For this review, take the finished solid that the model builds, in its own axes (mm). A direction names the side the tool comes from. Give positions to 0.01 mm unless a question says otherwise; leave off trailing zeros. Put each result on its own line as item: value. Start each with the question number.
from build123d import *

# Parameters (mm, degrees)
EXTRUDE_1_DEPTH                     = 401.066
SKETCH_2_R                          = 7.1501
CUT_EXTRUDE_1_DEPTH                 = 5.08
PATTERN_LINEAR_1_COUNT              = 8
PATTERN_LINEAR_1_PITCH              = 47.752
PATTERN_CIRCULAR_2_COUNT            = 3
PATTERN_CIRCULAR_2_ANGLE            = 180
PATTERN_CIRCULAR_2_COPY_1_SKETCH_R  = 7.1501
PATTERN_CIRCULAR_2_COPY_1_DEPTH     = 5.08
PATTERN_CIRCULAR_2_COPY_2_SKETCH_R  = 7.1501
PATTERN_CIRCULAR_2_COPY_2_DEPTH     = 5.08
PATTERN_CIRCULAR_2_COPY_3_SKETCH_R  = 7.1501
PATTERN_CIRCULAR_2_COPY_3_DEPTH     = 5.08
PATTERN_CIRCULAR_2_COPY_4_SKETCH_R  = 7.1501
PATTERN_CIRCULAR_2_COPY_4_DEPTH     = 5.08
PATTERN_CIRCULAR_2_COPY_5_SKETCH_R  = 7.1501
PATTERN_CIRCULAR_2_COPY_5_DEPTH     = 5.08
PATTERN_CIRCULAR_2_COPY_6_SKETCH_R  = 7.1501
PATTERN_CIRCULAR_2_COPY_6_DEPTH     = 5.08
PATTERN_CIRCULAR_2_COPY_7_SKETCH_R  = 7.1501
PATTERN_CIRCULAR_2_COPY_7_DEPTH     = 5.08
PATTERN_CIRCULAR_2_COPY_8_SKETCH_R  = 7.1501
PATTERN_CIRCULAR_2_COPY_8_DEPTH     = 5.08
PATTERN_CIRCULAR_2_COPY_9_SKETCH_R  = 7.1501
PATTERN_CIRCULAR_2_COPY_9_DEPTH     = 5.08
PATTERN_CIRCULAR_2_COPY_10_SKETCH_R = 7.1501
PATTERN_CIRCULAR_2_COPY_10_DEPTH    = 5.08
PATTERN_CIRCULAR_2_COPY_11_SKETCH_R = 7.1501
PATTERN_CIRCULAR_2_COPY_11_DEPTH    = 5.08
PATTERN_CIRCULAR_2_COPY_12_SKETCH_R = 7.1501
PATTERN_CIRCULAR_2_COPY_12_DEPTH    = 5.08
PATTERN_CIRCULAR_2_COPY_13_SKETCH_R = 7.1501
PATTERN_CIRCULAR_2_COPY_13_DEPTH    = 5.08
PATTERN_CIRCULAR_2_COPY_14_SKETCH_R = 7.1501
PATTERN_CIRCULAR_2_COPY_14_DEPTH    = 5.08


with BuildPart() as part:
    # 草图1 → 凸台-拉伸1 (new body)
    with BuildSketch(Plane.XY):
        with BuildLine():
            Line((0, 0), (35.98, 0))
            ThreePointArc((35.98, 0), (37.883814298, 0.788585702), (38.6724, 2.6924))
            Line((38.6724, 2.6924), (38.6724, 36.5252))
            ThreePointArc((38.6724, 36.5252), (33.8972, 41.3004), (29.122, 36.5252))
            ThreePointArc((29.122, 36.5252), (30.4682, 35.179), (31.8144, 36.5252))
            ThreePointArc((31.8144, 36.5252), (33.8972, 38.608), (35.98, 36.5252))
            Line((35.98, 36.5252), (35.98, 2.6924))
            Line((35.98, 2.6924), (0, 2.6924))
            Line((0, 2.6924), (0, 36.5252))
            ThreePointArc((0, 36.5252), (2.0828, 38.608), (4.1656, 36.5252))
            ThreePointArc((4.1656, 36.5252), (5.5118, 35.179), (6.858, 36.5252))
            ThreePointArc((6.858, 36.5252), (2.0828, 41.3004), (-2.6924, 36.5252))
            Line((-2.6924, 36.5252), (-2.6924, 2.6924))
            ThreePointArc((-2.6924, 2.6924), (-1.903814298, 0.788585702), (0, 0))
        make_face()
    extrude(amount=EXTRUDE_1_DEPTH)

    # 草图2 → 切除-拉伸1 (cut)
    with BuildSketch(Plane.ZY.offset(2.6924)):
        with Locations((24.6761, 19.6088)):
            Circle(SKETCH_2_R)
    cut_extrude_1 = extrude(amount=-CUT_EXTRUDE_1_DEPTH, mode=Mode.SUBTRACT)

    # 阵列(线性)1: 切除-拉伸1 ×8
    with Locations(*[(0, 0, i * PATTERN_LINEAR_1_PITCH) for i in range(1, PATTERN_LINEAR_1_COUNT)]):
        add(cut_extrude_1, mode=Mode.SUBTRACT)

    # 阵列(圆周)2: 切除-拉伸1 ×3 about axis
    pattern_circular_2_axis = Axis((17.99, 19.6088, 0), (0, 0, 1))
    for i in range(1, PATTERN_CIRCULAR_2_COUNT):
        add(cut_extrude_1.rotate(pattern_circular_2_axis, i * PATTERN_CIRCULAR_2_ANGLE / (PATTERN_CIRCULAR_2_COUNT - 1)), mode=Mode.SUBTRACT)

    # 阵列(圆周)2 copy 1 sketch → 阵列(圆周)2 copy 1 (cut)
    with BuildSketch(Plane(origin=(37.5988, -1.0736, 47.752), x_dir=(0, 0, 1), z_dir=(0, -1, 0))):
        with Locations((24.6761, 19.6088)):
            Circle(PATTERN_CIRCULAR_2_COPY_1_SKETCH_R)
    extrude(amount=-PATTERN_CIRCULAR_2_COPY_1_DEPTH, mode=Mode.SUBTRACT)

    # 阵列(圆周)2 copy 2 sketch → 阵列(圆周)2 copy 2 (cut)
    with BuildSketch(Plane(origin=(38.6724, 39.2176, 47.752), x_dir=(0, 0, 1), z_dir=(1, 0, 0))):
        with Locations((24.6761, 19.6088)):
            Circle(PATTERN_CIRCULAR_2_COPY_2_SKETCH_R)
    extrude(amount=-PATTERN_CIRCULAR_2_COPY_2_DEPTH, mode=Mode.SUBTRACT)

    # 阵列(圆周)2 copy 3 sketch → 阵列(圆周)2 copy 3 (cut)
    with BuildSketch(Plane(origin=(37.5988, -1.0736, 95.504), x_dir=(0, 0, 1), z_dir=(0, -1, 0))):
        with Locations((24.6761, 19.6088)):
            Circle(PATTERN_CIRCULAR_2_COPY_3_SKETCH_R)
    extrude(amount=-PATTERN_CIRCULAR_2_COPY_3_DEPTH, mode=Mode.SUBTRACT)

    # 阵列(圆周)2 copy 4 sketch → 阵列(圆周)2 copy 4 (cut)
    with BuildSketch(Plane(origin=(38.6724, 39.2176, 95.504), x_dir=(0, 0, 1), z_dir=(1, 0, 0))):
        with Locations((24.6761, 19.6088)):
            Circle(PATTERN_CIRCULAR_2_COPY_4_SKETCH_R)
    extrude(amount=-PATTERN_CIRCULAR_2_COPY_4_DEPTH, mode=Mode.SUBTRACT)

    # 阵列(圆周)2 copy 5 sketch → 阵列(圆周)2 copy 5 (cut)
    with BuildSketch(Plane(origin=(37.5988, -1.0736, 143.256), x_dir=(0, 0, 1), z_dir=(0, -1, 0))):
        with Locations((24.6761, 19.6088)):
            Circle(PATTERN_CIRCULAR_2_COPY_5_SKETCH_R)
    extrude(amount=-PATTERN_CIRCULAR_2_COPY_5_DEPTH, mode=Mode.SUBTRACT)

    # 阵列(圆周)2 copy 6 sketch → 阵列(圆周)2 copy 6 (cut)
    with BuildSketch(Plane(origin=(38.6724, 39.2176, 143.256), x_dir=(0, 0, 1), z_dir=(1, 0, 0))):
        with Locations((24.6761, 19.6088)):
            Circle(PATTERN_CIRCULAR_2_COPY_6_SKETCH_R)
    extrude(amount=-PATTERN_CIRCULAR_2_COPY_6_DEPTH, mode=Mode.SUBTRACT)

    # 阵列(圆周)2 copy 7 sketch → 阵列(圆周)2 copy 7 (cut)
    with BuildSketch(Plane(origin=(37.5988, -1.0736, 191.008), x_dir=(0, 0, 1), z_dir=(0, -1, 0))):
        with Locations((24.6761, 19.6088)):
            Circle(PATTERN_CIRCULAR_2_COPY_7_SKETCH_R)
    extrude(amount=-PATTERN_CIRCULAR_2_COPY_7_DEPTH, mode=Mode.SUBTRACT)

    # 阵列(圆周)2 copy 8 sketch → 阵列(圆周)2 copy 8 (cut)
    with BuildSketch(Plane(origin=(38.6724, 39.2176, 191.008), x_dir=(0, 0, 1), z_dir=(1, 0, 0))):
        with Locations((24.6761, 19.6088)):
            Circle(PATTERN_CIRCULAR_2_COPY_8_SKETCH_R)
    extrude(amount=-PATTERN_CIRCULAR_2_COPY_8_DEPTH, mode=Mode.SUBTRACT)

    # 阵列(圆周)2 copy 9 sketch → 阵列(圆周)2 copy 9 (cut)
    with BuildSketch(Plane(origin=(37.5988, -1.0736, 238.76), x_dir=(0, 0, 1), z_dir=(0, -1, 0))):
        with Locations((24.6761, 19.6088)):
            Circle(PATTERN_CIRCULAR_2_COPY_9_SKETCH_R)
    extrude(amount=-PATTERN_CIRCULAR_2_COPY_9_DEPTH, mode=Mode.SUBTRACT)

    # 阵列(圆周)2 copy 10 sketch → 阵列(圆周)2 copy 10 (cut)
    with BuildSketch(Plane(origin=(38.6724, 39.2176, 238.76), x_dir=(0, 0, 1), z_dir=(1, 0, 0))):
        with Locations((24.6761, 19.6088)):
            Circle(PATTERN_CIRCULAR_2_COPY_10_SKETCH_R)
    extrude(amount=-PATTERN_CIRCULAR_2_COPY_10_DEPTH, mode=Mode.SUBTRACT)

    # 阵列(圆周)2 copy 11 sketch → 阵列(圆周)2 copy 11 (cut)
    with BuildSketch(Plane(origin=(37.5988, -1.0736, 286.512), x_dir=(0, 0, 1), z_dir=(0, -1, 0))):
        with Locations((24.6761, 19.6088)):
            Circle(PATTERN_CIRCULAR_2_COPY_11_SKETCH_R)
    extrude(amount=-PATTERN_CIRCULAR_2_COPY_11_DEPTH, mode=Mode.SUBTRACT)

    # 阵列(圆周)2 copy 12 sketch → 阵列(圆周)2 copy 12 (cut)
    with BuildSketch(Plane(origin=(38.6724, 39.2176, 286.512), x_dir=(0, 0, 1), z_dir=(1, 0, 0))):
        with Locations((24.6761, 19.6088)):
            Circle(PATTERN_CIRCULAR_2_COPY_12_SKETCH_R)
    extrude(amount=-PATTERN_CIRCULAR_2_COPY_12_DEPTH, mode=Mode.SUBTRACT)

    # 阵列(圆周)2 copy 13 sketch → 阵列(圆周)2 copy 13 (cut)
    with BuildSketch(Plane(origin=(37.5988, -1.0736, 334.264), x_dir=(0, 0, 1), z_dir=(0, -1, 0))):
        with Locations((24.6761, 19.6088)):
            Circle(PATTERN_CIRCULAR_2_COPY_13_SKETCH_R)
    extrude(amount=-PATTERN_CIRCULAR_2_COPY_13_DEPTH, mode=Mode.SUBTRACT)

    # 阵列(圆周)2 copy 14 sketch → 阵列(圆周)2 copy 14 (cut)
    with BuildSketch(Plane(origin=(38.6724, 39.2176, 334.264), x_dir=(0, 0, 1), z_dir=(1, 0, 0))):
        with Locations((24.6761, 19.6088)):
            Circle(PATTERN_CIRCULAR_2_COPY_14_SKETCH_R)
    extrude(amount=-PATTERN_CIRCULAR_2_COPY_14_DEPTH, mode=Mode.SUBTRACT)


solid = part.part
1) Machinability: for faces 5 (the flat face through (0, 19, 198)), 6 (the cylindrical face through (37.35, 12.52, 23.75)), which of the approach directions +Z, -Z, +X, -X, +Y, -Y give a long, thin tool a straight path to every point of the face, cutting with its end or side? Answer none if there is none.
2) Mouldability with a two-part tool opening along X and no side actions: class faces 1 (the cylindrical face through (10.9, 1.33, 23.75)), 2 (the cylindrical face through (15.84, 1.33, 127)), 3 (the flat face through (-2.692, 20, 198)), 4 (the cylindrical face through (-1.37, 21.76, 174.75)) as released by +X, released by -X, zero draft, split by the parting line, or undercut.
3) Wall thickness on probe 1 along X at (y, z) = (6, 22); probe 2 along Y at (x, z) = (34, 142.5); probe 3 along Y at (x, z) = (24, 344.5): over which ranges is each line inside the solid? List them lowest first.
4) Take a section at B-B on x = 17.99. State how many separate pieces and enclosed holes the cut face has, and give its area (3 significant figures).
5) Insertion check: P1, Ø12, axis at x = 23, z = 245.5, coming from the +Y side. The pin has a flat end and moves straight along its axis. Give the tip position at first contact, or say it passes through.
Answers follow:
1. face 5: +Z, -Z
1. face 6: +X, -X
2. face 1: undercut
2. face 2: undercut
2. face 3: released by -X
2. face 4: zero draft
3. probe 1: -2.69 to 0, 35.98 to 38.67
3. probe 2: 0 to 2.69, 38.61 to 41.3
3. probe 3: 0 to 2.69
4. separate pieces: 9
4. enclosed holes: 0
4. area: 772 mm2
5. P1: y = 2.69
